from build123d import *

# Parameters (mm, degrees)
SKETCH_1_W              = 90
SKETCH_1_H              = 30
EXTRUDE_1_DEPTH         = 115
SKETCH_3_W              = 20
SKETCH_3_H              = 20
EXTRUDE_2_DEPTH         = 30
SKETCH_4_W              = 15
SKETCH_4_H              = 40
EXTRUDE_3_DEPTH         = 60
CUT_EXTRUDE_1_OUTLINE_R = 2
CUT_EXTRUDE_1_DEPTH     = 30


# Read off the part's stored shape, not the designer's step: 切除-拉伸1
with BuildPart() as part:
    # 草图1 → 凸台-拉伸1 (new body)
    with BuildSketch(Plane.XY):
        with Locations((0, 15)):
            Rectangle(SKETCH_1_W, SKETCH_1_H)
    extrude(amount=EXTRUDE_1_DEPTH)

    # 草图3 → 凸台-拉伸2 (add)
    with BuildSketch(Plane(origin=(45, 0, 0), x_dir=(0, 0, -1), z_dir=(1, 0, 0))):
        with Locations((-65, 20)):
            Rectangle(SKETCH_3_W, SKETCH_3_H)
    extrude(amount=EXTRUDE_2_DEPTH)

    # 草图4 → 凸台-拉伸3 (add)
    with BuildSketch(Plane(origin=(0, 30, 0), x_dir=(1, 0, 0), z_dir=(0, 1, 0))):
        with Locations((-37.5, -65)):
            Rectangle(SKETCH_4_W, SKETCH_4_H)
    extrude(amount=EXTRUDE_3_DEPTH)

    # 切除-拉伸1 outline → 切除-拉伸1 (cut)
    with BuildSketch(Plane(origin=(0, 0, 0), x_dir=(1, 0, 0), z_dir=(0, 1, 0))):
        with Locations((41.5, -4)):
            Circle(CUT_EXTRUDE_1_OUTLINE_R)
        with Locations((-36.9, -4)):
            Circle(CUT_EXTRUDE_1_OUTLINE_R)
        with Locations((-36.9, -111)):
            Circle(CUT_EXTRUDE_1_OUTLINE_R)
        with Locations((41.5, -111)):
            Circle(CUT_EXTRUDE_1_OUTLINE_R)
    extrude(amount=CUT_EXTRUDE_1_DEPTH, mode=Mode.SUBTRACT)


solid = part.part
CAD build for the part. Positions are in the model's coordinates, mm. A direction names the side the tool comes from. Round coordinates to 2 decimals unless told otherwise and drop trailing zeros. Write each loop counter-clockwise with the first axis right and the second up, starting at its lowest first coordinate (ties: lowest second). Pieces come first, ordered by that corner, then holes.
(1) Probe line 1 along Z through (x, y) = (41.5, 18.75); line 2 along X through (y, z) = (14.5, 4); line 3 along Y through (x, z) = (-9, 44). List the from-to ranges inside material, lowest first.
(2) Drop flat-ended pins along their axis: P1, Ø4.5, axis at x = -41, y = 48, coming from the +Z side; P2, Ø6, axis at x = 56.5, z = 65.5, coming from the -Y side; P3, Ø16.5, axis at x = -37.5, y = 58.5, coming from the -Z side. Give the stop position or say it passes through.
(3) 3-axis set-ups, long thin cutter, end or side, ignore diameter. For faces 1 (the face through (-38, 60, 85)), 2 (the face through (60, 20, 55)), 3 (the face through (60, 20, 75)): which of +Z, -Z, +X, -X, +Y, -Y reach the whole face in a straight line?
(4) Slice it at A-A, the plane z = 111. Write the cut outline in (x, y).
(5) Slice it at D-D, the plane z = 70. Write the cut outline in (x, y), and give its area (3 significant figures).
(6) Slice it at B-B, the plane x = 41.5. Write the cut outline in (y, z), and give its area (3 significant figures).
(7) Slice it at C-C, the plane y = 13. Write the cut outline in (x, z).
(8) Mould opens along X. For faces 4 (the face through (-30, 60, 65)), 5 (the face through (-38, 60, 45)), 6 (the face through (-35.053, 14.79, 4.766)) say: pulls with the +X half, pulls with the -X half, needs draft (parallel to the pull), parting line crosses it, or undercut.
From the geometry:
1. line 1: z = 0 to 2, 6 to 109, 113 to 115
1. line 2: x = -45 to -38.9, -34.9 to 39.5, 43.5 to 45
1. line 3: y = 0 to 30
2. P1: stops at z = 85
2. P2: stops at y = 10
2. P3: stops at z = 45
3. face 1: +Z, +X, -X, +Y
3. face 2: -Z, +X, +Y, -Y
3. face 3: +Z, +X, +Y, -Y
4. outline: (-45, 0) - (-38.9, 0) - (-38.9, 30) - (-45, 30) - close; (-34.9, 0) - (39.5, 0) - (39.5, 30) - (-34.9, 30) - close; (43.5, 0) - (45, 0) - (45, 30) - (43.5, 30) - close
5. outline: (-45, 0) - (45, 0) - (45, 10) - (75, 10) - (75, 30) - (-30, 30) - (-30, 90) - (-45, 90) - close
5. area: 4,200 mm2
6. outline: (0, 0) - (30, 0) - (30, 2) - (0, 2) - close; (0, 6) - (30, 6) - (30, 109) - (0, 109) - close; (0, 113) - (30, 113) - (30, 115) - (0, 115) - close
6. area: 3,210 mm2
7. outline: (-45, 0) - (45, 0) - (45, 55) - (75, 55) - (75, 75) - (45, 75) - (45, 115) - (-45, 115) - close; hole circle Ø4 at (-36.9, 4); hole circle Ø4 at (-36.9, 111); hole circle Ø4 at (41.5, 4); hole circle Ø4 at (41.5, 111)
8. face 4: pulls with the +X half
8. face 5: needs draft
8. face 6: undercut
